Work out the finished part from the listing and answer in its coordinate system (mm). Face numbers are marked on the shaded views. A direction names the side the tool comes from. Give positions to 0.01 mm unless a question says otherwise; leave off trailing zeros. Order: outer loops, then holes, each group sorted by start corner. A loop starts at its lowest first (then second) coordinate and runs counter-clockwise, first axis right, second up. Notation, with made-up numbers: (-0.75, -5.5) - (53.25, -5.5) arc R21 ccw to (53.25, 1.5) - close; hole circle Ø9 at (13.5, -3.75). An arc over 180 degrees is marked (long way). Write each question's results on one line, items separated by ' | '.
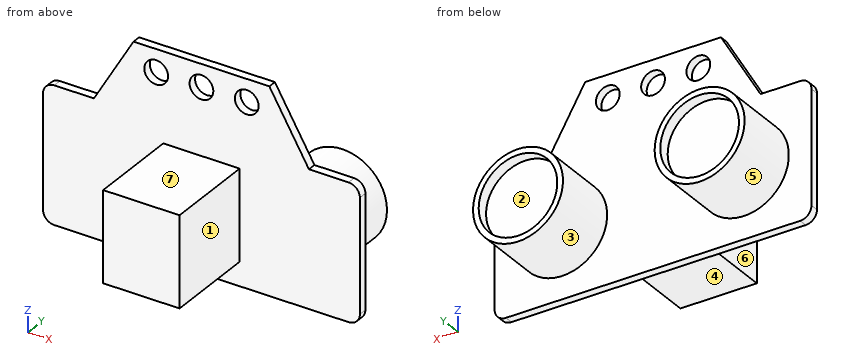
from build123d import *

# Parameters (mm, degrees)
SKETCH1_R           = 2.1
BOSS_EXTRUDE1_DEPTH = 1.5
FILLET1_R           = 2
SKETCH2_R           = 7.95
BOSS_EXTRUDE2_DEPTH = 12
SKETCH3_W           = 13.5
SKETCH3_H           = 16
BOSS_EXTRUDE3_DEPTH = 16.3
SKETCH4_R           = 6.95
CUT_EXTRUDE1_DEPTH  = 2


with BuildPart() as part:
    # Sketch1 → Boss-Extrude1 (new body)
    with BuildSketch(Plane(origin=(0, 0, 0), x_dir=(1, 0, 0), z_dir=(0, 1, 0))):
        Polygon((12, 0), (-12, 0), (-19, 12), (-28, 12), (-28, 36), (28, 36), (28, 12), (19, 12), align=None)
        with Locations((0, 4)):
            Circle(SKETCH1_R, mode=Mode.SUBTRACT)
        with Locations((-8, 4)):
            Circle(SKETCH1_R, mode=Mode.SUBTRACT)
        with Locations((8, 4)):
            Circle(SKETCH1_R, mode=Mode.SUBTRACT)
    extrude(amount=BOSS_EXTRUDE1_DEPTH)

    # Fillet1
    fillet1_edges = [part.edges().sort_by_distance(p)[0] for p in [
        (-28, 0.75, -12),
        (-28, 0.75, -36),
        (28, 0.75, -36),
        (28, 0.75, -12),
    ]]
    fillet(fillet1_edges, radius=FILLET1_R)

    # Sketch2 → Boss-Extrude2 (add)
    with BuildSketch(Plane(origin=(0, 1.5, 0), x_dir=(1, 0, 0), z_dir=(0, 1, 0))):
        with Locations((-16.05, 24.05)):
            Circle(SKETCH2_R)
        with Locations((16.05, 24.05)):
            Circle(SKETCH2_R)
    extrude(amount=BOSS_EXTRUDE2_DEPTH)

    # Sketch3 → Boss-Extrude3 (add)
    with BuildSketch(Plane.XZ):
        with Locations((0, -23.8)):
            Rectangle(SKETCH3_W, SKETCH3_H)
    extrude(amount=BOSS_EXTRUDE3_DEPTH)

    # Sketch4 → Cut-Extrude1 (cut)
    with BuildSketch(Plane(origin=(0, 13.5, 0), x_dir=(1, 0, 0), z_dir=(0, 1, 0))):
        with Locations((-16.05, 24.05)):
            Circle(SKETCH4_R)
        with Locations((16.05, 24.05)):
            Circle(SKETCH4_R)
    extrude(amount=-CUT_EXTRUDE1_DEPTH, mode=Mode.SUBTRACT)


solid = part.part
1. Given P1, Ø5, axis at y = -5.5, z = -21, coming from the -X side; P2, Ø8.5, axis at x = 16.05, z = -24.05, coming from the -Y side; P3, Ø2.5, axis at x = -8, z = -4, coming from the +Y side; P4, Ø7, axis at x = -3, y = -9.5, coming from the -Z side, each flat-ended and moving along its own axis, determine where each tip first touches the part or whether it passes through.
Answer list:
P1: x = -6.75 | P2: y = 0 | P3: through | P4: z = -31.8
2. A cutting plane is placed at C-C, the plane y = 8.25. Write down the section's boundary in (x, z).
Answer list:
outline: circle Ø15.9 at (-16.05, -24.05); circle Ø15.9 at (16.05, -24.05)
3. A tool of negligible diameter and unlimited length cuts with its end or side. For the marked faces 4, 5, 6 and 7, from which of +Z, -Z, +X, -X, +Y, -Y can it reach the whole face along a straight path? Write none if from no direction.
Answer list:
face 4: -Z, +X, -X, -Y | face 5: +Y | face 6: +Z, -Z, -X, -Y | face 7: +Z, +X, -X, -Y
4. A cutting plane is placed at D-D, the plane z = -20.5. Write down the section's boundary in (x, y).
Answer list:
outline: (-28, 0) - (-6.75, 0) - (-6.75, -16.3) - (6.75, -16.3) - (6.75, 0) - (28, 0) - (28, 1.5) - (23.16, 1.5) - (23.16, 13.5) - (22.02, 13.5) - (22.02, 11.5) - (10.08, 11.5) - (10.08, 13.5) - (8.94, 13.5) - (8.94, 1.5) - (-8.94, 1.5) - (-8.94, 13.5) - (-10.08, 13.5) - (-10.08, 11.5) - (-22.02, 11.5) - (-22.02, 13.5) - (-23.16, 13.5) - (-23.16, 1.5) - (-28, 1.5) - close
5. A cutting plane is placed at B-B, the plane z = -3. Write down the section's boundary in (x, y), then the cut area to 3 significant figures.
Answer list:
outline: (-13.75, 0) - (-9.85, 0) - (-9.85, 1.5) - (-13.75, 1.5) - close; (-6.15, 0) - (-1.85, 0) - (-1.85, 1.5) - (-6.15, 1.5) - close; (1.85, 0) - (6.15, 0) - (6.15, 1.5) - (1.85, 1.5) - close; (9.85, 0) - (13.75, 0) - (13.75, 1.5) - (9.85, 1.5) - close | area: 24.6 mm^2
6. Determine the mould class of the marked faces 1, 2 and 3 for opening direction Z: +Z half, -Z half, draft (parallel to the pull), parting line (faces both ways), or undercut.
Answer list:
face 1: draft | face 2: undercut | face 3: parting line
7. A cutting plane is placed at A-A, the plane x = 0. Write down the section's boundary in (y, z).
Answer list:
outline: (-16.3, -31.8) - (0, -31.8) - (0, -36) - (1.5, -36) - (1.5, -6.1) - (0, -6.1) - (0, -15.8) - (-16.3, -15.8) - close; (0, -1.9) - (1.5, -1.9) - (1.5, 0) - (0, 0) - close
8. Straight lines are drawn through the part: line 1 (X direction, y = 12.9, z = -24.05); line 2 (Z direction, x = 0, y = 0.3); line 3 (X direction, y = 0.9, z = -4). For each, find the intervals that lie inside material, in ascending order. Write a range as [from, to].
Answer list:
line 1: [-24, -23], [-9.1, -8.1], [8.1, 9.1], [23, 24] | line 2: [-36, -6.1], [-1.9, 0] | line 3: [-14.33, -10.1], [-5.9, -2.1], [2.1, 5.9], [10.1, 14.33]
